Part print with two shaded views. Sizes in mm from the minimum x, y, z corner. A direction names the side the tool comes from. Give positions to 0.01 mm unless a question says otherwise; leave off trailing zeros. Order: outer loops, then holes, each group sorted by start corner. A loop starts at its lowest first (then second) coordinate and runs counter-clockwise, first axis right, second up. Notation, with made-up numbers: M -1.75,28 L 28.25,28 A27 ccw 28.25,56 Z; hole C 50.5,33.5 d1. An arc over 180 degrees is marked long. Answer as CSV lines item,"result".
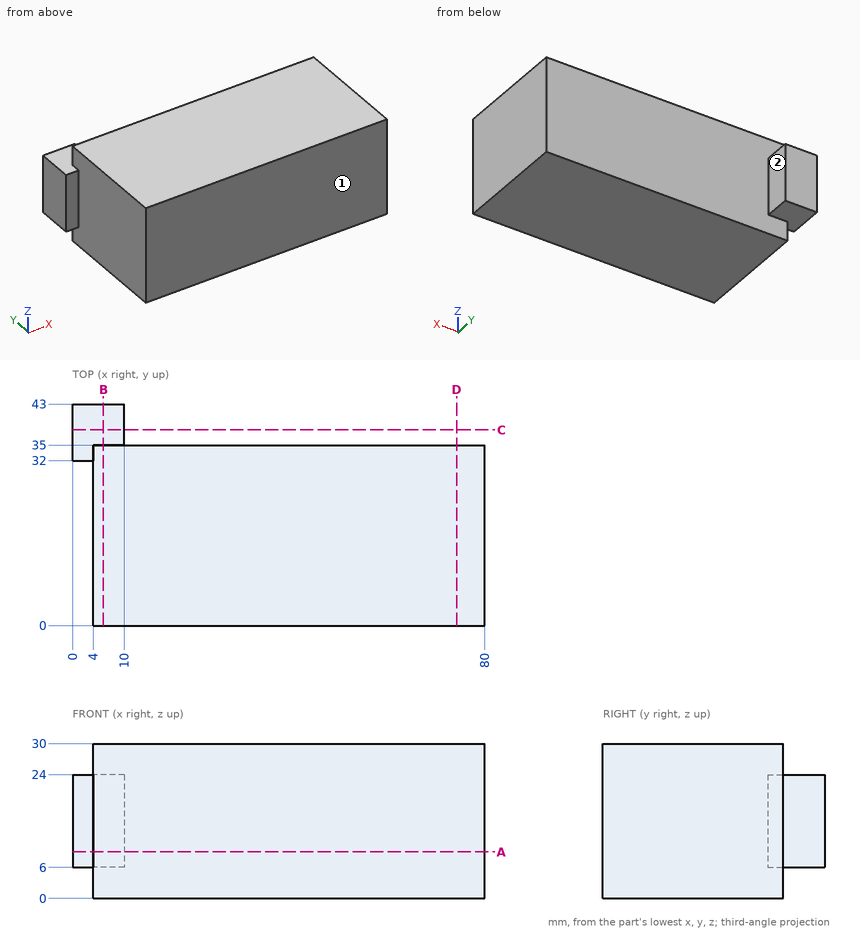
Item 1: Band-saw the part on C-C (y = 38). Give the cut face in (x, z), and give its area (3 significant figures).
Geometry says:
outline,"M 0,6 L 10,6 L 10,24 L 0,24 Z"
area,"180 mm2"
Item 2: Band-saw the part on B-B (x = 6). Give the cut face in (y, z), and give its area (3 significant figures).
Geometry says:
outline,"M 0,0 L 35,0 L 35,6 L 43,6 L 43,24 L 35,24 L 35,30 L 0,30 Z"
area,"1,190 mm2"
Item 3: 3-axis set-ups, long thin cutter, end or side, ignore diameter. For the marked faces 1 and 2: which of +Z, -Z, +X, -X, +Y, -Y reach the whole face in a straight line?
Geometry says:
face 1,"+Z, -Z, +X, -X, -Y"
face 2,"+Z, -Z, +X, +Y"
Item 4: Probe line 1 along X through (y, z) = (34.5, 27.5); line 2 along Y through (x, z) = (13.5, 3). List the from-to ranges inside material, lowest first. Write a range as from..to.
Geometry says:
line 1,"x = 4..80"
line 2,"y = 0..35"
Item 5: Band-saw the part on A-A (z = 9). Give the cut face in (x, y), and give its area (3 significant figures).
Geometry says:
outline,"M 0,32 L 4,32 L 4,0 L 80,0 L 80,35 L 10,35 L 10,43 L 0,43 Z"
area,"2,750 mm2"
Item 6: Drop flat-ended pins along their axis: pin 1 (9 mm diameter, centred on x = 29.5, z = 18, fed in from +Y); pin 2 (2 mm diameter, centred on x = 60, y = 15.5, fed in from -Z); pin 3 (2.5 mm diameter, centred on y = 40, z = 18.5, fed in from +X); pin 4 (1.5 mm diameter, centred on x = 26, y = 37, fed in from +Z). Give the stop position or say it passes through.
Geometry says:
pin 1,"stops at y = 35"
pin 2,"stops at z = 0"
pin 3,"stops at x = 10"
pin 4,"passes through"
Item 7: Band-saw the part on D-D (x = 74.5). Give the cut face in (y, z).
Geometry says:
outline,"M 0,0 L 35,0 L 35,30 L 0,30 Z"
